Autodesk Inventor part; units mm, degrees
ref_plane "YZ Plane" through (0, 0, 0) normal (1, 0, 0) x (0, 1, 0)
ref_plane "XZ Plane" through (0, 0, 0) normal (0, 1, 0) x (-1, 0, 0)
ref_plane "XY Plane" through (0, 0, 0) normal (0, 0, 1) x (1, 0, 0)
sketch "Sketch1" plane through (0, 0, 0) normal (0, 0, 1) x (1, 0, 0)
  line L0 (-11.7577, -18.2929) -> (28.2423, -18.2929)
  line L1 (28.2423, -18.2929) -> (28.2423, -3.2929)
  line L2 (28.2423, -3.2929) -> (-11.7577, -3.2929)
  line L3 (-11.7577, -3.2929) -> (-11.7577, -18.2929)
  point P0 (0, 0)
  dimension "d0" = 40
  dimension "d1" = 15
extrude "Extrusion1" add sketch "Sketch1" along normal blind 6
sketch "Sketch2" plane through (0, 0, 6) normal (0, 0, 1) x (1, 0, 0)
  line L0 (28.2423, -3.2929) -> (-11.7577, -3.2929)
  line L1 (15.2423, -3.2929) -> (15.2423, -18.2929)
  line L2 (1.2423, -3.2929) -> (1.2423, -18.2929)
  line L3 (-11.7577, -18.2929) -> (28.2423, -18.2929)
  line L4 (15.2423, -6.7382) -> (28.2423, -6.7382) construction
  line L5 (28.2423, -18.2929) -> (28.2423, -3.2929)
  line L6 (1.2423, -6.7382) -> (-11.7577, -6.7382) construction
  line L7 (-11.7577, -3.2929) -> (-11.7577, -18.2929)
  point P0 (0, 0)
  dimension "d4" = 14
extrude "Extrusion2" add sketch "Sketch2" along normal blind 25 contours L1 L3 L2 L0
sketch "Sketch4" plane through (0, 0, 6) normal (0, 0, 1) x (1, 0, 0)
  circle A0 centre (21.7423, -10.7929) radius 2.125
  line L0 (21.7423, -10.7929) -> (21.7423, -3.2929) construction
  line L1 (21.7423, -10.7929) -> (21.7423, -18.2929) construction
  line L2 (15.2423, -18.2929) -> (28.2423, -18.2929)
  line L3 (21.7423, -10.7929) -> (28.2423, -10.7929) construction
  line L4 (21.7423, -10.7929) -> (15.2423, -10.7929) construction
  line L5 (15.2423, -18.2929) -> (15.2423, -3.2929)
  line L6 (28.2423, -3.2929) -> (15.2423, -3.2929)
  line L7 (28.2423, -18.2929) -> (28.2423, -3.2929)
  circle A1 centre (-5.2577, -10.7929) radius 2.125
  line L8 (-5.2577, -10.7929) -> (-5.2577, -3.2929) construction
  line L9 (-5.2577, -10.7929) -> (-11.7577, -10.7929) construction
  line L10 (-11.7577, -3.2929) -> (-11.7577, -18.2929)
  line L11 (-5.2577, -10.7929) -> (-5.2577, -18.2929) construction
  line L12 (-5.2577, -10.7929) -> (1.2423, -10.7929) construction
  line L13 (1.2423, -3.2929) -> (1.2423, -18.2929)
  point P0 (0, 0)
  dimension "d12" = 4.25
  dimension "d13" = 4.25
extrude "Extrusion4" cut sketch "Sketch4" against normal up to next contours A0 | A1
sketch "Sketch5" plane through (1.2423, -18.2929, 6) normal (-1, 0, 0) x (0, 0, 1)
  circle A0 centre (10, 7.5) radius 4
  line L0 (10, 7.5) -> (10, 15) construction
  line L1 (10, 7.5) -> (10, 0) construction
  line L2 (-6, 15) -> (-6, 0)
  line L3 (13.9686, 7) -> (25, 7)
  line L4 (13.9686, 8) -> (25, 8)
  line L5 (25, 15) -> (25, 0)
  line L6 (27.4068, 8) -> (27.4068, 15) construction
  line L7 (27.4068, 7) -> (27.4068, 0) construction
  line L8 (0, 0) -> (25, 0)
  line L9 (0, 15) -> (25, 15)
  line L10 (10, 7.5) -> (10, 0) construction
  line L11 (0, 0) -> (25, 0)
  point P0 (-6, 18.2929)
  dimension "d16" = 8
  dimension "d17" = 16
  dimension "d18" = 1
extrude "Extrusion5" cut sketch "Sketch5" against normal up to next
sketch "Sketch6" plane through (-11.7577, -3.2929, 0) normal (0, 1, 0) x (1, 0, 0)
  circle A0 centre (20, -25) radius 2.125
  line L0 (27, -31) -> (13, -31)
  line L1 (20, -25) -> (27, -25) construction
  line L2 (20, -25) -> (13, -25) construction
  line L3 (27, -6) -> (27, -31)
  line L4 (13, -6) -> (13, -31)
  point P0 (11.7577, 0)
  dimension "d21" = 4.25
  dimension "d22" = 6
extrude "Extrusion6" cut sketch "Sketch6" against normal through all
sketch "Sketch7" plane through (-11.7577, -18.2929, 0) normal (0, -1, 0) x (1, 0, 0)
  circle A0 centre (20, 25) radius 2.125
  circle A1 centre (20, 25) radius 5
  point P0 (11.7577, 0)
  dimension "d25" = 10
sketch "Sketch8" plane through (-11.7577, -18.2929, 0) normal (0, -1, 0) x (1, 0, 0)
  circle A0 centre (15.7148, 27.4964) radius 1.6
  circle A1 centre (15.7148, 8.4964) radius 1.6
  circle A2 centre (15.7148, 27.4964) radius 1.6
  circle A3 centre (15.7148, 8.4964) radius 1.6
  point P0 (11.7577, 0)
extrude "Extrusion8" cut sketch "Sketch8" against normal up to next contours A0
extrude "Extrusion9" cut sketch "Sketch8" against normal up to surface (15 mm away) contours A1
sketch "Sketch9" plane through (0, 0, 31) normal (0, 0, 1) x (1, 0, 0)
  point P0 (0, 0)
sketch "Sketch10" plane through (1.2423, -11.2929, 31) normal (0, 1, 0) x (1, 0, 0)
  line L0 (6, 6) -> (6, 0)
  line L1 (14, 0) -> (0, 0)
  line L2 (6, 0) -> (0, 0)
  line L3 (0, 11.0314) -> (14, 11.0314)
  line L4 (0, 11.0314) -> (0, 19)
  line L5 (6, 6) -> (0, 6)
  line L6 (0, 0) -> (0, 11.0314)
  line L7 (0, 0) -> (0, 6)
  point P0 (-1.2423, 31)
  dimension "d32" = 6
  dimension "d35" = 6
extrude "Extrusion10" cut sketch "Sketch10" against normal blind 1.5
properties part number "YRodClampWithEndstop"
Model file for the job. Use its own axes, mm. A direction names the side the tool comes from. Give positions to 0.01 mm unless a question says otherwise; leave off trailing zeros. Loops run counter-clockwise (first coordinate to the right, second up) from the corner with the lowest first, then second, coordinate; pieces in that order, holes last.
1) Pull direction Y, two halves, no side cores. Call faces 1 (the cylindrical face through (3.61, -10.898, 6.934)), 2 (the flat face through (7.242, -12, 29)), 3 (the flat face through (8, -18.293, 12)): +Y half, -Y half, draft (parallel to the pull), parting line (faces both ways), or undercut.
2) Wall check: line 1 (X direction, y = -17.5, z = 25); line 2 (Z direction, x = 7, y = -7.75); line 3 (Z direction, x = 3, y = -7.25). Give the ranges that are in metal, low to high.
3) Saw through at D-D (y = -15.75). Write the cut outline in (x, z) (3 decimals), plus the area to 3 significant figures.
4) Saw through at A-A (z = 9). Write the cut outline in (x, y).
5) Tool access for faces 4 (the flat face through (20, -9, 6)), 5 (the flat face through (-7, -9, 6)), 6 (the flat face through (4.2, -12.793, 29.3)): list every direction of +Z, -Z, +X, -X, +Y, -Y with a clear straight run to the whole face (end or side of a thin tool).
6) Flat gauge pins, fed straight in: pin 1 Ø6.5 at (x, y) = (20.5, -9.5) entering from +Z; pin 2 Ø2.5 at (x, z) = (3.96, 27.5) entering from -Y. Where does each tip first touch, or does it go through?
7) Saw through at B-B (z = 23.5). Write the cut outline in (x, y).
8) Saw through at C-C (x = 22.5). Write the cut outline in (y, z), plus the area to 3 significant figures.
Answer block:
1. face 1: draft
1. face 2: undercut
1. face 3: -Y half
2. line 1: x = 1.24 to 6.12, 10.37 to 15.24
2. line 2: z = 0 to 13.4, 18.6 to 23.28, 26.72 to 31
2. line 3: z = 0 to 7.21, 9.78 to 14.14, 17.86 to 31
3. outline: (-11.758, 0) - (28.242, 0) - (28.242, 6) - (15.242, 6) - (15.242, 31) - (1.242, 31) - (1.242, 6) - (-11.758, 6) - close; hole circle Ø3.2 at (3.957, 8.496); hole circle Ø3.2 at (3.957, 27.496); hole circle Ø4.25 at (8.242, 25)
3. area: 560 mm2
4. outline: (1.24, -18.29) - (2.44, -18.29) - (2.44, -3.29) - (1.24, -3.29) - close; (5.48, -18.29) - (15.24, -18.29) - (15.24, -3.29) - (5.48, -3.29) - close
5. face 4: +Z, +X, +Y, -Y
5. face 5: +Z, -X, +Y, -Y
5. face 6: +Z, -X
6. pin 1: stops at z = 6
6. pin 2: stops at y = -10.29
7. outline: (1.24, -18.29) - (6.74, -18.29) - (6.74, -11.29) - (1.24, -11.29) - close; (1.24, -10.29) - (6.74, -10.29) - (6.74, -3.29) - (1.24, -3.29) - close; (9.75, -18.29) - (15.24, -18.29) - (15.24, -11.29) - (9.75, -11.29) - close; (9.75, -10.29) - (15.24, -10.29) - (15.24, -3.29) - (9.75, -3.29) - close
8. outline: (-18.29, 0) - (-12.78, 0) - (-12.78, 6) - (-18.29, 6) - close; (-8.81, 0) - (-3.29, 0) - (-3.29, 6) - (-8.81, 6) - close
8. area: 66.2 mm2
